```python
from build123d import *

# Parameters (mm, degrees)
SKETCH1_R            = 2.7499999999999987
BOSS_EXTRUDE1_DEPTH  = 2.5
BOSS_EXTRUDE3_DEPTH  = 4.25
SKETCH5_R            = 1.4999999999999967
CUT_EXTRUDE1_DEPTH   = 5
FILLET1_R            = 1
FILLET2_R            = 1
FILLET3_R            = 1
FILLET4_R            = 1
FILLET1_OF_MIRROR1_R = 1
FILLET2_OF_MIRROR1_R = 1
FILLET3_OF_MIRROR1_R = 1
FILLET4_OF_MIRROR1_R = 1
FILLET5_R            = 5
FILLET6_R            = 5


with BuildPart() as part:
    # Sketch1 → Boss-Extrude1 (new body)
    with BuildSketch(Plane(origin=(0, 0, 0), x_dir=(1, 0, 0), z_dir=(0, 1, 0))):
        Polygon((0, 0), (-30, 0), (-45, -5.51e-15), (-45, -30), (-29.999999999999996, -30), (-30, -42), (-15, -42), (-15, -30.000000000000004), (0, -30), align=None)
        with Locations(Location((-22.5, -37.239999999999995, 0), (0, 0, 270))):
            Circle(SKETCH1_R, mode=Mode.SUBTRACT)
        with BuildLine():
            Line((-34.99999999999999, -1.239999999999998), (-10.000000000000002, -1.240000000000011))
            ThreePointArc((-10.000000000000002, -1.240000000000011), (-7.500000000000012, -3.7400000000000007), (-10.000000000000002, -6.2399999999999896))
            Line((-10.000000000000002, -6.2399999999999896), (-34.99999999999999, -6.240000000000009))
            ThreePointArc((-34.99999999999999, -6.240000000000009), (-37.5, -3.7400000000000015), (-34.99999999999999, -1.239999999999998))
        make_face(mode=Mode.SUBTRACT)
        with BuildLine():
            Line((-34.99999999999999, -23.75999999999999), (-10.000000000000002, -23.76000000000001))
            ThreePointArc((-10.000000000000002, -23.76000000000001), (-7.500000000000012, -26.259999999999998), (-10.000000000000002, -28.759999999999987))
            Line((-10.000000000000002, -28.759999999999987), (-34.99999999999999, -28.76))
            ThreePointArc((-34.99999999999999, -28.76), (-37.5, -26.259999999999998), (-34.99999999999999, -23.75999999999999))
        make_face(mode=Mode.SUBTRACT)
    extrude(amount=BOSS_EXTRUDE1_DEPTH)

    # Sketch3 → Boss-Extrude3 (add, symmetric)
    with BuildSketch(Plane.XY.offset(14.999999999999995)):
        Polygon((-39.5, 2.5), (-42.5, 2.5000000000000004), (-42.5, 12), (-42.5, 15.000000000000007), (-34.5, 15.000000000000004), (-34.5, 12), (-39.5, 12), align=None)
    boss_extrude3 = extrude(amount=BOSS_EXTRUDE3_DEPTH, both=True)

    # Sketch5 → Cut-Extrude1 (cut)
    with BuildSketch(Plane(origin=(6.51e-15, 14.999999999999988, 0), x_dir=(1, 0, 0), z_dir=(0, 1, 0))):
        with Locations(Location((-36.99999999999999, -15, 0), (0, 0, 270))):
            Circle(SKETCH5_R)
    cut_extrude1 = extrude(amount=-CUT_EXTRUDE1_DEPTH, mode=Mode.SUBTRACT)

    # Fillet1
    fillet1_edges = [part.edges().sort_by_distance(p)[0] for p in [
        (-39.49999999999999, 12, 14.999999999999993),
    ]]
    fillet(fillet1_edges, radius=FILLET1_R)

    # Fillet2
    fillet2_edges = [part.edges().sort_by_distance(p)[0] for p in [
        (-34.49999999999999, 12, 14.999999999999993),
    ]]
    fillet(fillet2_edges, radius=FILLET2_R - 0.0001)  # a hair under: the kernel refuses the full size

    # Fillet3
    fillet3_edges = [part.edges().sort_by_distance(p)[0] for p in [
        (-34.49999999999999, 15.000000000000004, 14.999999999999993),
    ]]
    fillet(fillet3_edges, radius=FILLET3_R - 0.0001)  # a hair under: the kernel refuses the full size

    # Fillet4
    fillet4_edges = [part.edges().sort_by_distance(p)[0] for p in [
        (-42.49999999999999, 15.000000000000007, 14.999999999999993),
    ]]
    fillet(fillet4_edges, radius=FILLET4_R)

    # Mirror1: Boss-Extrude3, Cut-Extrude1 across plane
    add(boss_extrude3.mirror(Plane(origin=(-22.5, 0, 0), x_dir=(6e-17, 0, 1), z_dir=(1, 0, -6e-17))))
    add(cut_extrude1.mirror(Plane(origin=(-22.5, 0, 0), x_dir=(6e-17, 0, 1), z_dir=(1, 0, -6e-17))), mode=Mode.SUBTRACT)

    # Fillet1 of Mirror1
    fillet1_of_mirror1_edges = [part.edges().sort_by_distance(p)[0] for p in [
        (-5.500000000000007, 12, 14.999999999999991),
    ]]
    fillet(fillet1_of_mirror1_edges, radius=FILLET1_OF_MIRROR1_R)

    # Fillet2 of Mirror1
    fillet2_of_mirror1_edges = [part.edges().sort_by_distance(p)[0] for p in [
        (-10.500000000000007, 12, 14.999999999999993),
    ]]
    fillet(fillet2_of_mirror1_edges, radius=FILLET2_OF_MIRROR1_R - 0.0001)  # a hair under: the kernel refuses the full size

    # Fillet3 of Mirror1
    fillet3_of_mirror1_edges = [part.edges().sort_by_distance(p)[0] for p in [
        (-10.500000000000007, 15.000000000000004, 14.999999999999993),
    ]]
    fillet(fillet3_of_mirror1_edges, radius=FILLET3_OF_MIRROR1_R - 0.0001)  # a hair under: the kernel refuses the full size

    # Fillet4 of Mirror1
    fillet4_of_mirror1_edges = [part.edges().sort_by_distance(p)[0] for p in [
        (-2.500000000000007, 15.000000000000007, 14.999999999999991),
    ]]
    fillet(fillet4_of_mirror1_edges, radius=FILLET4_OF_MIRROR1_R)

    # Fillet5
    fillet5_edges = [part.edges().sort_by_distance(p)[0] for p in [
        (-15, 1.25, 30.000000000000004),
        (-29.999999999999996, 1.25, 30),
    ]]
    fillet(fillet5_edges, radius=FILLET5_R)

    # Fillet6
    fillet6_edges = [part.edges().sort_by_distance(p)[0] for p in [
        (0, 1.25, 30),
        (-15, 1.25, 42),
        (-30, 1.25, 42),
        (-45, 1.25, 30),
        (-45, 1.25, 5.51e-15),
        (0, 1.25, 0),
    ]]
    fillet(fillet6_edges, radius=FILLET6_R)


solid = part.part
```
Could you check a few things on this model? Use its own coordinates, in mm. A direction names the side the tool comes from. Coordinates: 2 decimals unless noted, no trailing zeros. Write each loop counter-clockwise with the first axis right and the second up, starting at its lowest first coordinate (ties: lowest second). Pieces come first, ordered by that corner, then holes. Notation, with made-up numbers: (64.5, 37) - (108.5, 37) arc R20 cw to (108.5, 66) - close; hole circle Ø6 at (46, 16.5). An arc over 180 degrees is marked (long way). Use a Markdown table: item, result.
Q1. Thinking about a two-plate mould opening in Y: for faces 4 (the cylindrical face through (-10.215, 14.699, 14.94)), 5 (the cylindrical face through (-36.93, 13.52, 13.5)), 6 (the flat face through (-39.5, 7, 15)), 7 (the flat face through (-5.5, 7, 15)), which applies, +Y half, -Y half, draft (parallel to the pull), parting line (faces both ways), or undercut?
Geometry check:
| item | result |
|---|---|
| face 4 | +Y half |
| face 5 | draft |
| face 6 | undercut |
| face 7 | undercut |
Q2. Imagine slicing it at A-A (x = -22.5). List the corners of the cut face in (y, z) for me.
Geometry check:
| item | result |
|---|---|
| outline | (0, 0) - (2.5, 0) - (2.5, 1.24) - (0, 1.24) - close; (0, 6.24) - (2.5, 6.24) - (2.5, 23.76) - (0, 23.76) - close; (0, 28.76) - (2.5, 28.76) - (2.5, 34.49) - (0, 34.49) - close; (0, 39.99) - (2.5, 39.99) - (2.5, 42) - (0, 42) - close |
Q3. Which directions (+Z, -Z, +X, -X, +Y, -Y) give clear straight access to the entire face, cutting with the end or side of a thin tool? Please do faces 1 (the cylindrical face through (-34.785, 14.699, 14.94)), 2 (the flat face through (-2.5, 8, 15)), 3 (the cylindrical face through (-37.5, 1.2, 26.3)).
Geometry check:
| item | result |
|---|---|
| face 1 | +Z, -Z, +Y |
| face 2 | +Z, -Z, +X, +Y |
| face 3 | +Y, -Y |
Q4. Imagine slicing it at B-B (x = -13). List the corners of the cut face in (y, z) for me, and give its area (3 significant figures).
Geometry check:
| item | result |
|---|---|
| outline | (0, 0) - (2.5, 0) - (2.5, 1.24) - (0, 1.24) - close; (0, 6.24) - (2.5, 6.24) - (2.5, 23.76) - (0, 23.76) - close; (0, 28.76) - (2.5, 28.76) - (2.5, 31) - (0, 31) - close |
| area | 52.5 mm2 |
Q5. Please list where these lines run through material, in increasing order: L1, parallel to X at y = 13.4, z = 15; L2, parallel to X at y = 9.5, z = 17.5; L3, parallel to Z at x = -8, y = 13.9.
Geometry check:
| item | result |
|---|---|
| L1 | x = -42.5 to -38.5, -35.5 to -34.5, -10.5 to -9.5, -6.5 to -2.5 |
| L2 | x = -42.5 to -39.5, -5.5 to -2.5 |
| L3 | z = 10.75 to 13.5, 16.5 to 19.25 |
Q6. I'm going to push flat-ended pins straight in: pin 1 Ø0.5 at (y, z) = (13.5, 15.5) entering from +X; pin 2 Ø4 at (x, z) = (-19.5, 9.5) entering from +Y; pin 3 Ø3 at (x, y) = (-38, 1.5) entering from +Z. Where does each tip first touch, or does it pass through?
Geometry check:
| item | result |
|---|---|
| pin 1 | stops at x = -2.5 |
| pin 2 | stops at y = 2.5 |
| pin 3 | stops at z = 30 |
Q7. Imagine slicing it at C-C (y = 1.25). List the corners of the cut face in (x, z) for me.
Geometry check:
| item | result |
|---|---|
| outline | (-45, 5) arc R5 ccw to (-40, 0) - (-5, 0) arc R5 ccw to (0, 5) - (0, 25) arc R5 ccw to (-5, 30) - (-10, 30) arc R5 cw to (-15, 35) - (-15, 37) arc R5 ccw to (-20, 42) - (-25, 42) arc R5 ccw to (-30, 37) - (-30, 35) arc R5 cw to (-35, 30) - (-40, 30) arc R5 ccw to (-45, 25) - close; hole (-35, 1.24) - (-10, 1.24) arc R2.5 ccw to (-10, 6.24) - (-35, 6.24) arc R2.5 ccw to start; hole (-35, 23.76) - (-10, 23.76) arc R2.5 ccw to (-10, 28.76) - (-35, 28.76) arc R2.5 ccw to start; hole circle Ø5.5 at (-22.5, 37.24) |
Q8. Imagine slicing it at D-D (y = 8.25). List the corners of the cut face in (x, z) for me.
Geometry check:
| item | result |
|---|---|
| outline | (-42.5, 10.75) - (-39.5, 10.75) - (-39.5, 19.25) - (-42.5, 19.25) - close; (-5.5, 10.75) - (-2.5, 10.75) - (-2.5, 19.25) - (-5.5, 19.25) - close |
